Source: three-view drawing plus pictorial views. Frame: mm from the lowest corner of the part. A direction names the side the tool comes from. Coordinates: 2 decimals unless noted, no trailing zeros. Order: outer loops, then holes, each group sorted by start corner. A loop starts at its lowest first (then second) coordinate and runs counter-clockwise, first axis right, second up. Notation, with made-up numbers: M 61.25,-21 L 101.25,-21 A14 cw 101.25,0 Z; hole C 13,19.5 d3. An arc over 180 degrees is marked long. Write item = value, one per line. Start each with the question number.
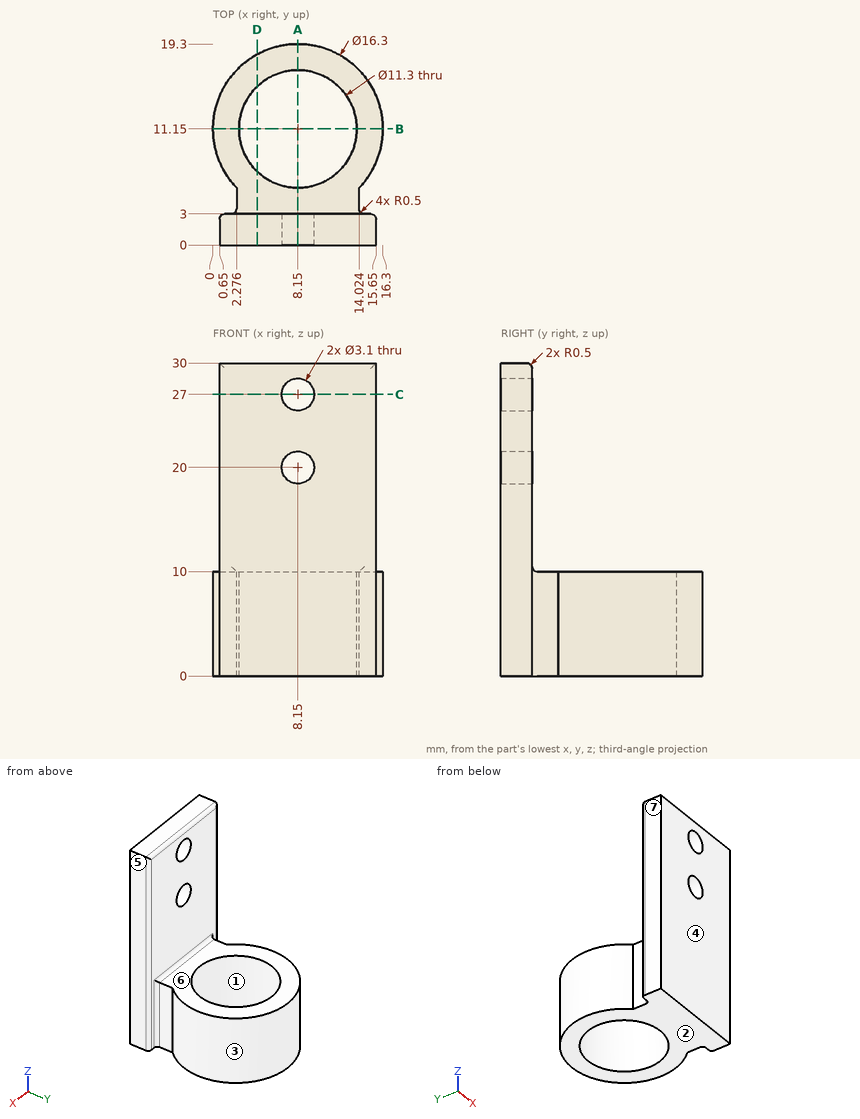
Item 1: Section query D-D on x = 4.25. Output: boundary loops of the cut face in (y, z), and give its area (3 significant figures).
Item 2: Material intervals for probe 1 along Z at (x, y) = (8.15, 0.75); probe 2 along X at (y, z) = (11.15, 7.25); probe 3 along Z at (x, y) = (15.5, 12), sorted ascending. Write a range as [from, to].
Item 3: Section query A-A on x = 8.15. Output: boundary loops of the cut face in (y, z).
Item 4: Reachability of the marked faces 5, 6 and 7 from +Z, -Z, +X, -X, +Y, -Y: full face, straight path, thin tool, end or side. Return the list, or none.
Item 5: Section query B-B on y = 11.15. Output: boundary loops of the cut face in (x, z), and give its area (3 significant figures).
Item 6: Section query C-C on z = 27. Output: boundary loops of the cut face in (x, y).
Item 7: Draft query along Y for the marked faces 1, 2, 3 and 4. Return one class per face: pulls with the +Y half, pulls with the -Y half, needs draft (parallel to the pull), parting line crosses it, or undercut.
Item 8: First-contact query: pin 1 (1.5 mm diameter, centred on x = 11, z = 23, fed in from +Y); pin 2 (3 mm diameter, centred on y = 1, z = 22, fed in from -X); pin 3 (6 mm diameter, centred on y = 17, z = 7.5, fed in from +X) (1 decimal); pin 4 (7 mm diameter, centred on x = 8.15, y = 11.15, fed in from +Z). Flat tips, straight axial feed; report the tip coordinate or a pass-through.
Ans:
q1.outline = M 0,0 L 7.06,0 L 7.06,10 L 3.5,10 A0.5 cw 3,10.5 L 3,29.5 A0.5 ccw 2.5,30 L 0,30 Z; M 15.24,0 L 18.31,0 L 18.31,10 L 15.24,10 Z
q1.area = 161 mm^2
q2.probe_1 = [0, 18.45], [21.55, 25.45], [28.55, 30]
q2.probe_2 = [0, 2.5], [13.8, 16.3]
q2.probe_3 = [0, 10]
q3.outline = M 0,0 L 5.5,0 L 5.5,10 L 3.5,10 A0.5 cw 3,10.5 L 3,18.45 L 0,18.45 Z; M 0,21.55 L 3,21.55 L 3,25.45 L 0,25.45 Z; M 0,28.55 L 3,28.55 L 3,29.5 A0.5 ccw 2.5,30 L 0,30 Z; M 16.8,0 L 19.3,0 L 19.3,10 L 16.8,10 Z
q4.face_5 = +Z, -Z, +X, -Y
q4.face_6 = +Z, +X, -X, +Y
q4.face_7 = +Z, -Z, -X, -Y
q5.outline = M 0,0 L 2.5,0 L 2.5,10 L 0,10 Z; M 13.8,0 L 16.3,0 L 16.3,10 L 13.8,10 Z
q5.area = 50.0 mm^2
q6.outline = M 0.65,0 L 6.6,0 L 6.6,3 L 1.15,3 A0.5 ccw 0.65,2.5 Z; M 9.7,0 L 15.65,0 L 15.65,2.5 A0.5 ccw 15.15,3 L 9.7,3 Z
q7.face_1 = undercut
q7.face_2 = needs draft
q7.face_3 = undercut
q7.face_4 = pulls with the -Y half
q8.pin_1 = 3
q8.pin_2 = 0.65
q8.pin_3 = 15.8
q8.pin_4 = through
